from build123d import *

# Parameters (mm, degrees)
SKETCH1_W           = 209.55
SKETCH1_H           = 25.4
BOSS_EXTRUDE1_DEPTH = 2.286
SKETCH2_R           = 3.96875
CUT_EXTRUDE1_DEPTH  = 3.286


with BuildPart() as part:
    # Sketch1 → Boss-Extrude1 (new body)
    with BuildSketch(Plane(origin=(0, 0, 0), x_dir=(1, 0, 0), z_dir=(0, 1, 0))):
        with Locations((104.775, 12.7)):
            Rectangle(SKETCH1_W, SKETCH1_H)
    extrude(amount=BOSS_EXTRUDE1_DEPTH)

    # Sketch2 → Cut-Extrude1 (cut, through all)
    with BuildSketch(Plane(origin=(0, 2.286, 0), x_dir=(1, 0, 0), z_dir=(0, 1, 0))):
        with Locations((196.85, 12.7)):
            Circle(SKETCH2_R)
        with BuildLine():
            Line((10.2, 14.358312395), (10.2, 11.041687605))
            ThreePointArc((10.2, 11.041687605), (15.7, 12.7), (10.2, 14.358312395))
        make_face()
    extrude(amount=-CUT_EXTRUDE1_DEPTH, mode=Mode.SUBTRACT)


solid = part.part
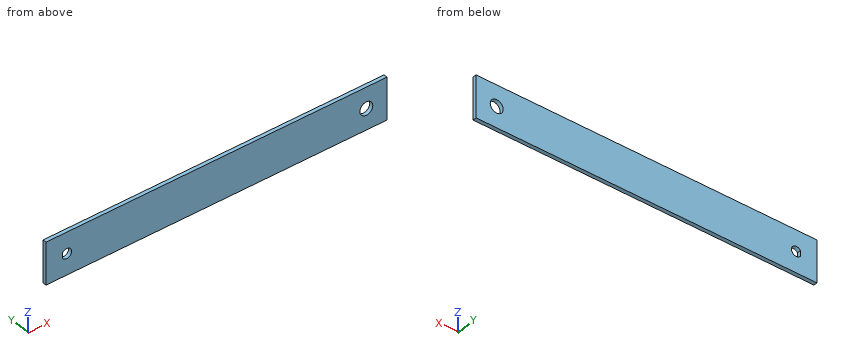
Input: part model. Units: mm. Frame: model coordinates. Give positions to 0.01 mm unless a question says otherwise; leave off trailing zeros. Loops run counter-clockwise (first coordinate to the right, second up) from the corner with the lowest first, then second, coordinate; pieces in that order, holes last. Notation, with made-up numbers: M -31,-37 L -16,-37 A20 cw -16,-27 Z; hole C -30,58.25 d1. An arc over 180 degrees is marked long. Use one line per item in the form item = value.
1. Line query: L1, parallel to X at y = 1, z = -12.7; L2, parallel to Z at x = 196.85, y = 1.65; L3, parallel to Z at x = 12.7, y = 0.6. Output: solid intervals per line, ascending.
Numbers:
L1 = 0 to 10.2, 15.7 to 192.88, 200.82 to 209.55
L2 = -25.4 to -16.67, -8.73 to 0
L3 = -25.4 to -15.7, -9.7 to 0
2. Section query B-B, the plane x = 12.7. Return the cut outline in (y, z).
Numbers:
outline = M 0,-25.4 L 2.29,-25.4 L 2.29,-15.7 L 0,-15.7 Z; M 0,-9.7 L 2.29,-9.7 L 2.29,0 L 0,0 Z
3. Section query A-A, the plane x = 196.85. Return the cut outline in (y, z), and give its area (3 significant figures).
Numbers:
outline = M 0,-25.4 L 2.29,-25.4 L 2.29,-16.67 L 0,-16.67 Z; M 0,-8.73 L 2.29,-8.73 L 2.29,0 L 0,0 Z
area = 39.9 mm²
